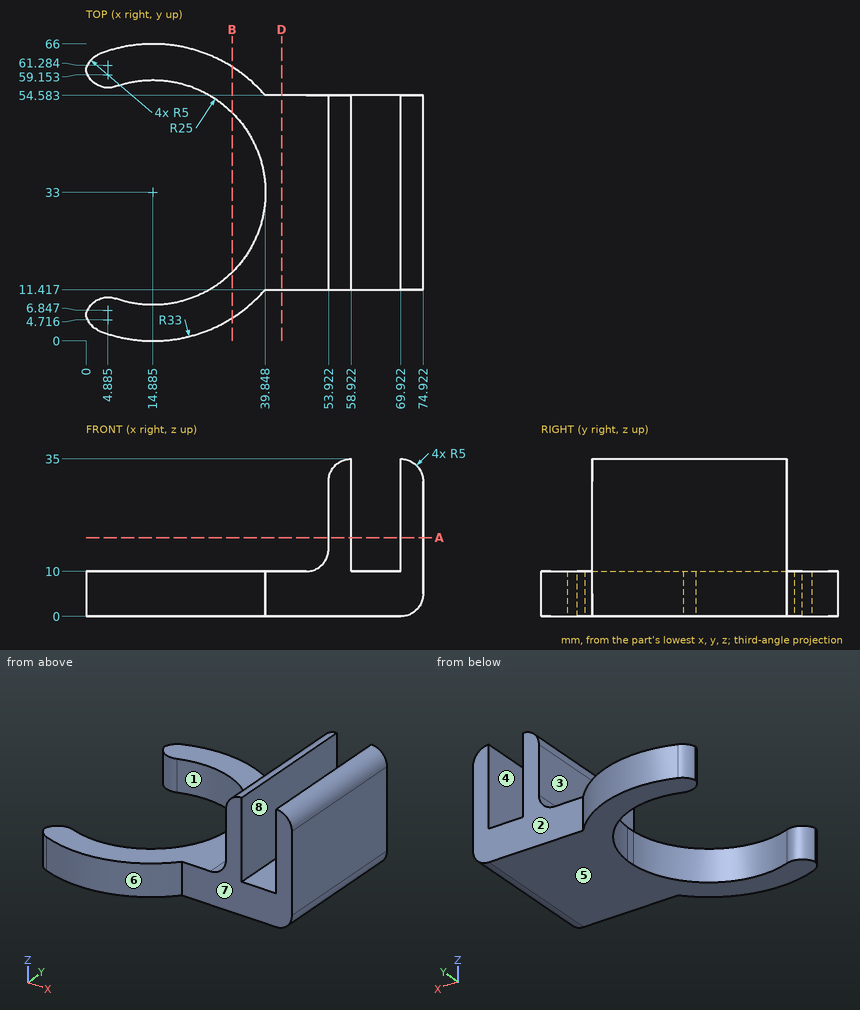
Job drawing, mm, ordinate dimensions from the low corner. One solid piece. A direction names the side the tool comes from. Coordinates: 2 decimals unless noted, no trailing zeros. Write each loop counter-clockwise with the first axis right and the second up, starting at its lowest first coordinate (ties: lowest second). Pieces come first, ordered by that corner, then holes. Notation, with made-up numbers: M 19,50 L 45,50 A21 cw 45,89 Z; hole C -29.5,42 d7. An arc over 180 degrees is marked long. Answer as a JSON object with one key per item and string values. Group by question number.
1) Tool access for the marked faces 1, 2, 3, 4 and 5: list every direction of +Z, -Z, +X, -X, +Y, -Y with a clear straight run to the whole face (end or side of a thin tool).
2) Wall check: line 1 (X direction, y = 17.5, z = 26); line 2 (Y direction, x = 55.5, z = 24); line 3 (Z direction, x = 68.5, y = 47.5). Give the ranges that are in metal, low to high. Write a range as from..to.
3) Saw through at A-A (z = 17.5). Write the cut outline in (x, y).
4) Pin check, flat tips, straight feed: pin 1 Ø3 at (y, z) = (50.5, 20.5) entering from -X; pin 2 Ø2 at (x, z) = (18.5, 10.5) entering from +Y (1 decimal); pin 3 Ø2 at (y, z) = (33, 6.5) entering from -X. Stop position of each tip, or through.
5) Mould opens along X. For the marked faces 6, 7 and 8 say: +X half, -X half, draft (parallel to the pull), parting line (faces both ways), or undercut.
6) Saw through at D-D (x = 43.5). Write the cut outline in (y, z), plus the area to 3 significant figures.
7) Saw through at B-B (x = 32.5). Write the cut outline in (y, z) (1 decimal), plus the area to 3 significant figures.
Values follow:
{
 "1": {"face 1": "+Z, -Z", "face 2": "+Z, -Z, +X, +Y", "face 3": "+Z, -X, +Y, -Y", "face 4": "+Z, +Y, -Y", "face 5": "-Z, +X, -X, +Y, -Y"},
 "2": {"line 1": "x = 53.92..58.92, 69.92..74.92", "line 2": "y = 11.42..54.58", "line 3": "z = 0..10"},
 "3": {"outline": "M 53.92,11.42 L 58.92,11.42 L 58.92,54.58 L 53.92,54.58 Z; M 69.92,11.42 L 74.92,11.42 L 74.92,54.58 L 69.92,54.58 Z"},
 "4": {"pin 1": "stops at x = 53.92", "pin 2": "stops at y = 65.9", "pin 3": "stops at x = 39.85"},
 "5": {"face 6": "parting line", "face 7": "draft", "face 8": "undercut"},
 "6": {"outline": "M 11.42,0 L 54.58,0 L 54.58,10 L 11.42,10 Z", "area": "432 mm2"},
 "7": {"outline": "M 5.1,0 L 15.3,0 L 15.3,10 L 5.1,10 Z; M 50.7,0 L 60.9,0 L 60.9,10 L 50.7,10 Z", "area": "203 mm2"}
}
